The model under review builds one solid part; all positions refer to its coordinate system, in mm. A direction names the side the tool comes from. Round coordinates to 2 decimals unless told otherwise and drop trailing zeros. Write each loop counter-clockwise with the first axis right and the second up, starting at its lowest first coordinate (ties: lowest second). Pieces come first, ordered by that corner, then holes. Notation, with made-up numbers: M 69.25,44 L 118.25,44 A7 cw 118.25,56 Z; hole C -9,58 d10. An arc over 180 degrees is marked long. One line per item, written item: value. Start each with the question number.
1) Wall thickness on probe 1 along X at (y, z) = (-35, 0.1); probe 2 along X at (y, z) = (-72, 1.45); probe 3 along Y at (x, z) = (4, 0.9): over which ranges is each line inside the solid? List them lowest first.
2) Take a section at C-C, the plane x = 6.75. Write out the cut boundary in (y, z).
3) Tool access review of faces 1 (the face through (25.6, -70.5, -0.7)), 2 (the face through (14, -68, -1.5)), 3 (the face through (20.95, -7.75, 1.48)), 4 (the face through (4, -69, -1)): name each direction out of +Z, -Z, +X, -X, +Y, -Y from which nothing blocks a thin tool from reaching the whole face with its end or side.
4) For P1, Ø6, axis at x = 5, y = -40.5, coming from the -Z side, flat-tipped, find the tip position at first contact; note if it passes through.
5) Take a section at B-B, the plane x = 16.75. Write out the cut boundary in (y, z), and give its area (3 significant figures).
6) Take a section at A-A, the plane y = -51.5. Write out the cut boundary in (x, z).
from build123d import *

# Parameters (mm, degrees)
F0_R     = 1.8
F1_DEPTH = 3
F3_DEPTH = 27
F4_DEPTH = 27
F5_DEPTH = 1.5


with BuildPart() as f1:
    # F0 (on Top) → F1 (new body)
    with BuildSketch(Plane.XY):
        Polygon((27, 0), (0, 0), (0, -75), (2.2679491924, -75), (0.5358983849, -72), (2.2679491924, -69), (5.7320508076, -69), (7.4641016151, -72), (5.7320508076, -75), (21.2679491924, -75), (19.5358983849, -72), (21.2679491924, -69), (24.7320508076, -69), (26.4641016151, -72), (24.7320508076, -75), (27, -75), align=None)
        with BuildLine():
            Line((3.75, -55), (3.75, -10))
            ThreePointArc((3.75, -10), (6, -7.75), (8.25, -10))
            Line((8.25, -10), (8.25, -55))
            ThreePointArc((8.25, -55), (6, -57.25), (3.75, -55))
        make_face(mode=Mode.SUBTRACT)
        with BuildLine():
            Line((18.75, -55), (18.75, -10))
            ThreePointArc((18.75, -10), (21, -7.75), (23.25, -10))
            Line((23.25, -10), (23.25, -55))
            ThreePointArc((23.25, -55), (21, -57.25), (18.75, -55))
        make_face(mode=Mode.SUBTRACT)
        Polygon((21.2679491924, -75), (24.7320508076, -75), (26.4641016151, -72), (24.7320508076, -69), (21.2679491924, -69), (19.5358983849, -72), align=None)
        with Locations((23, -72)):
            Circle(F0_R, mode=Mode.SUBTRACT)
        Polygon((0.5358983849, -72), (2.2679491924, -75), (5.7320508076, -75), (7.4641016151, -72), (5.7320508076, -69), (2.2679491924, -69), align=None)
        with Locations((4, -72)):
            Circle(F0_R, mode=Mode.SUBTRACT)
    extrude(amount=F1_DEPTH)

    # F2 (on face) → F3 (cut, through all)
    with BuildSketch(Plane.YZ.offset(27)):
        with BuildLine():
            Line((-65, 3), (-68, 3))
            ThreePointArc((-68, 3), (-66.5, 1.5), (-65, 3))
        make_face()
    extrude(amount=-F3_DEPTH, mode=Mode.SUBTRACT)

    # F2 (on face) → F4 (join, through all)
    with BuildSketch(Plane.YZ.offset(27)):
        Polygon((-59, 0), (-75, 0), (-75, -1.5), (-60.5, -1.5), align=None)
    extrude(amount=-F4_DEPTH)

    # F0 (on Top) → F5 (cut, through all)
    with BuildSketch(Plane.XY):
        Polygon((0.5358983849, -72), (2.2679491924, -75), (5.7320508076, -75), (7.4641016151, -72), (5.7320508076, -69), (2.2679491924, -69), align=None)
        with Locations((4, -72)):
            Circle(F0_R, mode=Mode.SUBTRACT)
        Polygon((21.2679491924, -75), (24.7320508076, -75), (26.4641016151, -72), (24.7320508076, -69), (21.2679491924, -69), (19.5358983849, -72), align=None)
        with Locations((23, -72)):
            Circle(F0_R, mode=Mode.SUBTRACT)
        with Locations((4, -72)):
            Circle(F0_R)
        with Locations((23, -72)):
            Circle(F0_R)
    extrude(amount=-F5_DEPTH, mode=Mode.SUBTRACT)


solid = f1.part
Checked values:
1. probe 1: x = 0 to 3.75, 8.25 to 18.75, 23.25 to 27
1. probe 2: x = 0 to 2.2, 5.8 to 21.2, 24.8 to 27
1. probe 3: y = -75 to -73.8, -70.2 to -56.03, -8.97 to 0
2. outline: M -75,-1.5 L -73.24,-1.5 L -73.24,0 L -70.76,0 L -70.76,-1.5 L -60.5,-1.5 L -59,0 L -57.12,0 L -57.12,3 L -65,3 A1.5 cw -68,3 L -75,3 Z; M -7.88,0 L 0,0 L 0,3 L -7.88,3 Z
3. face 1: -Z
3. face 2: -Z, +X, -X, +Y, -Y
3. face 3: +Z, -Z
3. face 4: -Z, -Y
4. P1: stops at z = 0
5. outline: M -75,-1.5 L -60.5,-1.5 L -59,0 L 0,0 L 0,3 L -65,3 A1.5 cw -68,3 L -75,3 Z
5. area: 244 mm2
6. outline: M 0,0 L 3.75,0 L 3.75,3 L 0,3 Z; M 8.25,0 L 18.75,0 L 18.75,3 L 8.25,3 Z; M 23.25,0 L 27,0 L 27,3 L 23.25,3 Z
